Could you check a few things on this drawing? It's one solid part, dimensions in mm from its lowest x, y, z. Give positions to 0.01 mm unless a question says otherwise; leave off trailing zeros. Order: outer loops, then holes, each group sorted by start corner. A loop starts at its lowest first (then second) coordinate and runs counter-clockwise, first axis right, second up.
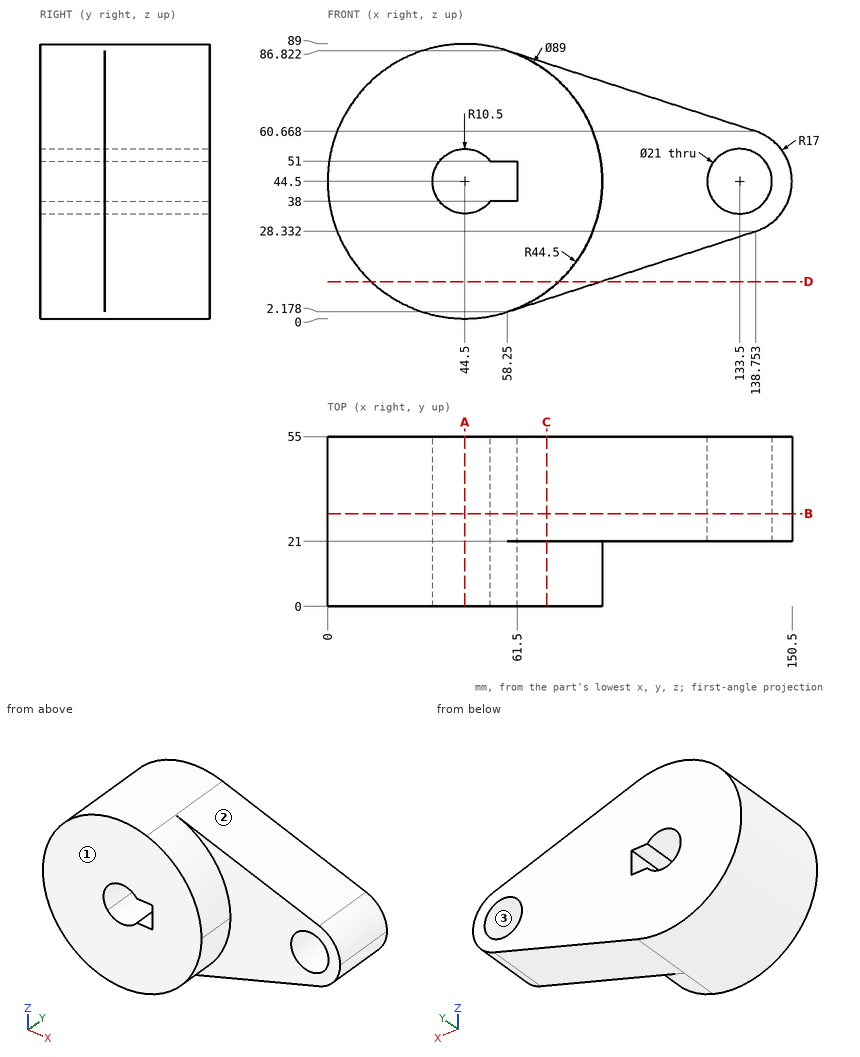
Item 1: Please list where these lines run through material, in increasing order: line 1 along X through (y, z) = (28, 44); line 2 along X through (y, z) = (32, 39.5); line 3 along Y through (x, z) = (103.5, 59.5).
Findings:
line 1: x = 0 to 34.01, 61.5 to 123.01, 143.99 to 150.49
line 2: x = 0.28 to 35.27, 61.5 to 124.27, 142.73 to 149.75
line 3: y = 21 to 55
Item 2: We'd pull the mould along X, two halves only. Please class the marked faces 1, 2 and 3: +X half, -X half, draft (parallel to the pull), parting line (faces both ways), or undercut.
Findings:
face 1: draft
face 2: +X half
face 3: undercut
Item 3: For pin 1 (2.5 mm diameter, centred on x = 55, y = 25, fed in from -Z); pin 2 (12 mm diameter, centred on x = 133.5, z = 31.5, fed in from -Y); pin 3 (9.5 mm diameter, centred on x = 57, y = 36.5, fed in from +Z), each with a flat end and sliding along its axis, tell me the tip position at first contact or that it passes through.
Findings:
pin 1: stops at z = 0.97
pin 2: stops at y = 21
pin 3: stops at z = 88.32
Item 4: Imagine slicing it at A-A on x = 44.5. List the corners of the cut face in (y, z) for me, then the cut area to 3 significant figures.
Findings:
outline: (0, 0) - (55, 0) - (55, 34) - (0, 34) - close; (0, 55) - (55, 55) - (55, 89) - (0, 89) - close
area: 3,740 mm2
Item 5: Imagine slicing it at D-D on z = 12. List the corners of the cut face in (x, y) for me, then the cut area to 3 significant figures.
Findings:
outline: (14.1, 0) - (74.9, 0) - (74.9, 21) - (88.48, 21) - (88.48, 55) - (14.1, 55) - close
area: 3,810 mm2
Item 6: Imagine slicing it at C-C on x = 71. List the corners of the cut face in (y, z) for me.
Findings:
outline: (0, 8.75) - (21, 8.75) - (21, 6.32) - (55, 6.32) - (55, 82.68) - (21, 82.68) - (21, 80.25) - (0, 80.25) - close
Item 7: Imagine slicing it at B-B on y = 30. List the corners of the cut face in (x, z) for me.
Findings:
outline: (58.25, 2.18) - (138.75, 28.33) arc R17 ccw to (138.75, 60.67) - (58.25, 86.82) arc R44.5 ccw (long way) to start; hole (52.75, 38) - (61.5, 38) - (61.5, 51) - (52.75, 51) arc R10.5 ccw (long way) to start; hole circle Ø21 at (133.5, 44.5)
